Geometry check sheet. Reference: the model listing, model coordinates, mm. A direction names the side the tool comes from. Give positions to 0.01 mm unless a question says otherwise; leave off trailing zeros. Loops run counter-clockwise (first coordinate to the right, second up) from the corner with the lowest first, then second, coordinate; pieces in that order, holes last.
1. Release check for a two-part mould opening along Z. For faces 1 (the flat face through (1, 18, 7.056)), 2 (the cylindrical face through (0.986, -0.542, -16.615)), 3 (the flat face through (1, 0, -34.056)), 4 (the flat face through (1, 10, -21)) record: +Z half, -Z half, draft (parallel to the pull), parting line (faces both ways), or undercut.
2. Cross-section at C-C, the plane x = 1.4. Record the cut outline in (y, z).
3. Cross-section at A-A, the plane y = 0. Record the cut outline in (x, z).
4. Go/stop test with flat-tipped pins: pin 1 Ø1 at (x, y) = (1, 38) entering from +Z; pin 2 Ø1 at (x, z) = (1, 19) entering from +Y; pin 3 Ø1 at (x, y) = (1.5, 6.5) entering from +Z. Record where each tip stops, or that it passes through.
5. Material ranges on L1, parallel to Z at x = 1.3, y = 0; L2, parallel to Y at x = 1.95, z = 28; L3, parallel to Z at x = 1.4, y = 29, recorded low to high.
6. Tool access check on faces 5 (the flat face through (1, 0, 34.056)), 6 (the flat face through (1, 26, -7.056)), 7 (the flat face through (1, 10, 20)). Record the directions out of +Z, -Z, +X, -X, +Y, -Y that give a thin tool (end or side, any length) a straight path to the whole face; none if there is none.
7. Cross-section at B-B, the plane z = 11. Record the cut outline in (x, y).
8. Cross-section at D-D, the plane y = 28.5. Record the cut outline in (x, z), plus the area to 3 significant figures.
Autodesk Inventor part; units mm, degrees
ref_plane "YZ Plane" through (0, 0, 0) normal (1, 0, 0) x (0, 1, 0)
ref_plane "XZ Plane" through (0, 0, 0) normal (0, 1, 0) x (-1, 0, 0)
ref_plane "XY Plane" through (0, 0, 0) normal (0, 0, 1) x (1, 0, 0)
sketch "Sketch1" plane through (0, 0, 0) normal (1, 0, 0) x (0, 1, 0)
  line L0 (10, 34.056) -> (-10, 34.056)
  line L1 (-10, 34.056) -> (-10, -34.056)
  line L2 (-10, -34.056) -> (10, -34.056)
  line L3 (10, -34.056) -> (10, 34.056)
  line L4 (10, 34.056) -> (-10, -34.056) construction
  line L5 (-10, 34.056) -> (10, -34.056) construction
  line L6 (10, 0) -> (10, -7.056)
  line L7 (10, -7.056) -> (42, -7.056)
  line L8 (42, -7.056) -> (42, 7.056)
  line L9 (42, 7.056) -> (10, 7.056)
  line L10 (10, 7.056) -> (10, -7.056)
  line L11 (0, 34.056) -> (0, 19.056)
  line L12 (0, -34.056) -> (0, -19.056)
  circle A0 centre (0, 19.056) radius 2.5
  circle A1 centre (0, -19.056) radius 2.5
  line L13 (10, 7.056) -> (10, 34.056)
  line L14 (10, 7.056) -> (10, 19.9232)
  line L15 (10, 19.9232) -> (25, 19.9232)
  line L16 (25, 19.9232) -> (25, 7.056)
  line L17 (25, 7.056) -> (10, 7.056)
  line L18 (25, 7.056) -> (25, 71.168)
  line L19 (25, 71.168) -> (35, 71.168)
  line L20 (35, 71.168) -> (35, 7.056)
  line L21 (35, 7.056) -> (25, 7.056)
  line L22 (35, 7.056) -> (35, 27.056)
  line L23 (35, 27.056) -> (25, 27.056)
  line L24 (35, 71.168) -> (35, 57.168)
  line L25 (35, 57.168) -> (25, 57.168)
  point P0 (0, 0)
  point P1 (0, 0)
  dimension "d0" = 20
  dimension "d1" = 68.112
  dimension "d2" = 7.056
  dimension "d3" = 32
  dimension "d4" = 14.112
  dimension "d5" = 15
  dimension "d6" = 15
  dimension "d7" = 5
  dimension "d8" = 5
  dimension "d9" = 15
  dimension "d10" = 64.112
  dimension "d11" = 10
  dimension "d12" = 20
  dimension "d13" = 14
extrude "Extrusion1" add sketch "Sketch1" along normal blind 2 contours L3 L2 L1 L0 | L9 L8 L7 L3 | L18 L23 L20 L9 L16 | L18 L25 L20 L23 | L18 L19 L20 L25
properties part number "manual_locker_raw"
Result:
1. face 1: +Z half
1. face 2: undercut
1. face 3: -Z half
1. face 4: draft
2. outline: (-10, -34.06) - (10, -34.06) - (10, -7.06) - (42, -7.06) - (42, 7.06) - (35, 7.06) - (35, 71.17) - (25, 71.17) - (25, 7.06) - (10, 7.06) - (10, 34.06) - (-10, 34.06) - close; hole circle Ø5 at (0, -19.06); hole circle Ø5 at (0, 19.06)
3. outline: (0, -34.06) - (2, -34.06) - (2, -21.56) - (0, -21.56) - close; (0, -16.56) - (2, -16.56) - (2, 16.56) - (0, 16.56) - close; (0, 21.56) - (2, 21.56) - (2, 34.06) - (0, 34.06) - close
4. pin 1: stops at z = 7.06
4. pin 2: stops at y = 35
4. pin 3: stops at z = 34.06
5. L1: z = -34.06 to -21.56, -16.56 to 16.56, 21.56 to 34.06
5. L2: y = -10 to 10, 25 to 35
5. L3: z = -7.06 to 71.17
6. face 5: +Z, +X, -X, -Y
6. face 6: -Z, +X, -X, +Y
6. face 7: +Z, +X, -X
7. outline: (0, -10) - (2, -10) - (2, 10) - (0, 10) - close; (0, 25) - (2, 25) - (2, 35) - (0, 35) - close
8. outline: (0, -7.06) - (2, -7.06) - (2, 71.17) - (0, 71.17) - close
8. area: 156 mm2
